Study the drawing (mm; zero at the part's minimum x, y, z) and answer. A direction names the side the tool comes from. Round coordinates to 2 decimals unless told otherwise and drop trailing zeros. Order: outer loops, then holes, each group sorted by start corner. A loop starts at its lowest first (then second) coordinate and runs counter-clockwise, first axis right, second up. Notation, with made-up numbers: M 65.25,-32.5 L 84.25,-32.5 A13 ccw 84.25,-9.5 Z; hole C 39.5,60.25 d8. An arc over 180 degrees is marked long. Put each result on its own line as item: value. Start each with the question number.
1. Consider line 1 (X direction, y = 0.8, z = 49.36); line 2 (X direction, y = 11.5, z = 44); line 3 (Z direction, x = 21.5, y = 2) (1 decimal). Determine where each line is inside the solid, lowest interval first.
2. The part is cut by section A-A (z = 13.36). Give the vertices of the cut face in (x, y).
3. Which of the six approach directions +Z, -Z, +X, -X, +Y, -Y give full straight-line access (tool end or side, diameter ignored) to the marked faces 3 and 4?
4. The mould has two halves that part along Z. Classify the marked faces 1 and 2: +Z half, -Z half, draft (parallel to the pull), parting line (faces both ways), or undercut.
5. The part is cut by section C-C (z = 46.5). Give the vertices of the cut face in (x, y).
6. The part is cut by section B-B (y = 6.75). Give the vertices of the cut face in (x, z) (1 decimal).
7. The part is cut by section D-D (y = 1). Count the separate pieces of the cut face and the enclosed holes in it, then the cut area to 3 significant figures.
8. Each of these flat-tipped pins is pushed along its axis until it touches: pin 1 Ø3.5 at (x, y) = (16.5, 2) entering from -Z; pin 2 Ø0.9 at (y, z) = (2.5, 61) entering from +X; pin 3 Ø3.5 at (x, z) = (10.56, 13.36) entering from +Y; pin 4 Ø6 at (x, y) = (14.5, 8) entering from -Z. Where does it stop, or does it pass through?
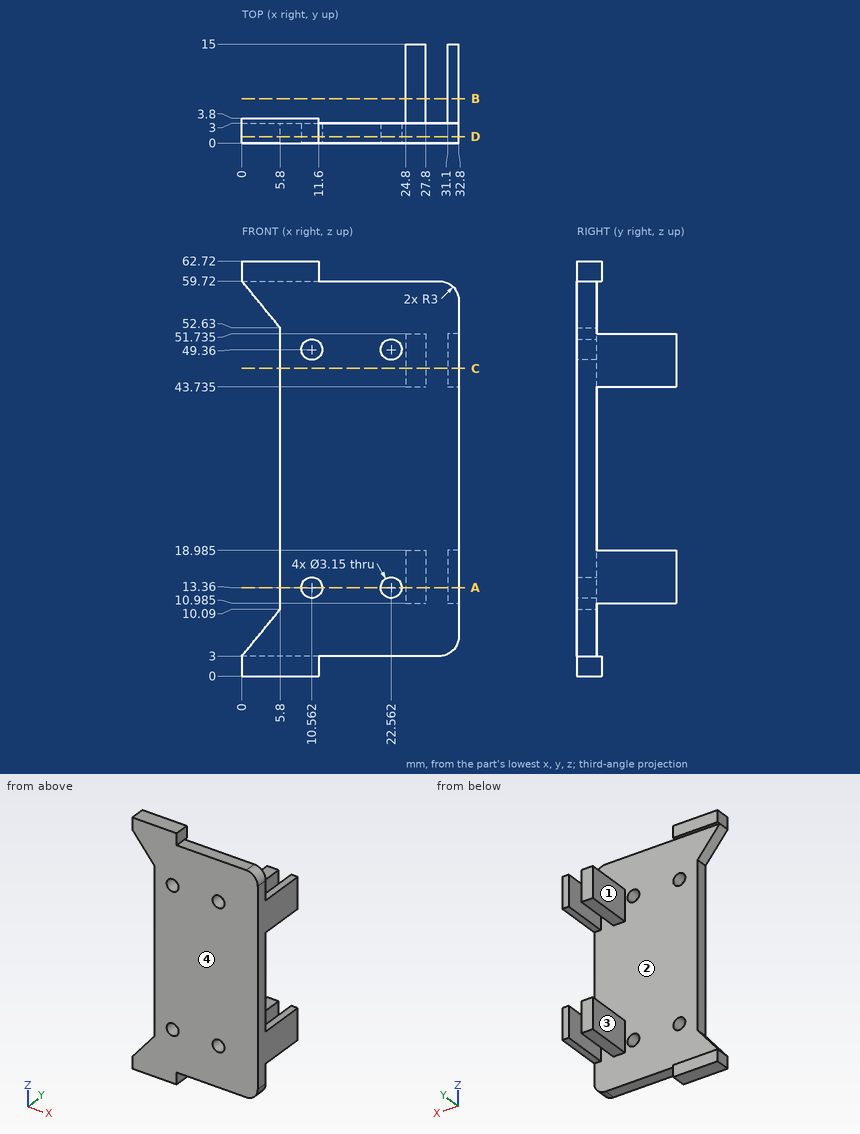
Resolved:
1. line 1: 5.8 to 8.99, 12.14 to 20.99, 24.14 to 32.8
1. line 2: 24.8 to 27.8, 31.1 to 32.8
1. line 3: 3 to 12.2, 14.5 to 48.2, 50.5 to 59.7
2. outline: M 5.8,0 L 8.99,0 L 8.99,3 L 5.8,3 Z; M 12.14,0 L 20.99,0 L 20.99,3 L 12.14,3 Z; M 24.14,0 L 32.8,0 L 32.8,15 L 31.1,15 L 31.1,3 L 27.8,3 L 27.8,15 L 24.8,15 L 24.8,3 L 24.14,3 Z
3. face 3: +Z, -Z, -X, +Y
3. face 4: +Z, -Z, +X, -X, -Y
4. face 1: draft
4. face 2: undercut
5. outline: M 5.8,0 L 32.8,0 L 32.8,15 L 31.1,15 L 31.1,3 L 27.8,3 L 27.8,15 L 24.8,15 L 24.8,3 L 5.8,3 Z
6. outline: M 24.8,11 L 27.8,11 L 27.8,19 L 24.8,19 Z; M 24.8,43.7 L 27.8,43.7 L 27.8,51.7 L 24.8,51.7 Z; M 31.1,11 L 32.8,11 L 32.8,19 L 31.1,19 Z; M 31.1,43.7 L 32.8,43.7 L 32.8,51.7 L 31.1,51.7 Z
7. separate pieces: 1
7. enclosed holes: 4
7. area: 1,610 mm2
8. pin 1: z = 3
8. pin 2: x = 11.6
8. pin 3: y = 3
8. pin 4: through
